For this review, take the finished solid that the model builds, in its own axes (mm). Face numbers are marked on the shaded views. Give positions to 0.01 mm unless a question says otherwise; leave off trailing zeros. Loops run counter-clockwise (first coordinate to the right, second up) from the corner with the lowest first, then second, coordinate; pieces in that order, holes last.
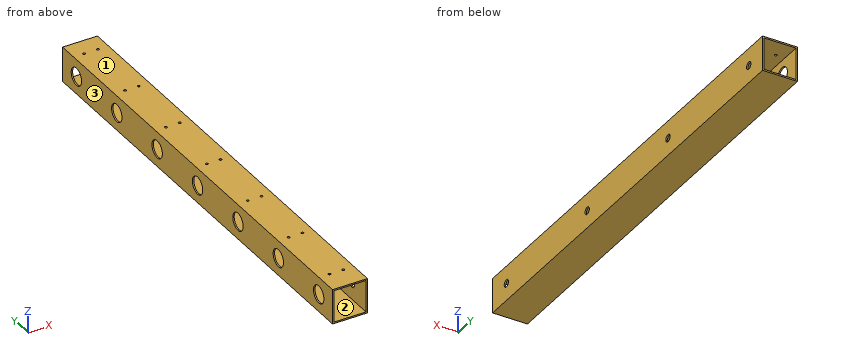
```python
from build123d import *

# Parameters (mm, degrees)
F0_W     = 76.2
F0_H     = 76.2
F0_W_2   = 69.85
F0_H_2   = 69.85
F1_DEPTH = 990.6
F2_R     = 2.75
F3_DEPTH = 25.4
F4_R     = 7.9375
F5_DEPTH = 25.4
F6_R     = 19.05
F7_DEPTH = 25.4


with BuildPart() as f1:
    # F0 (on Front) → F1 (new body)
    with BuildSketch(Plane.XZ):
        Rectangle(F0_W, F0_H)
        Rectangle(F0_W_2, F0_H_2, mode=Mode.SUBTRACT)
    extrude(amount=F1_DEPTH)

    # F2 (on face) → F3 (cut)
    with BuildSketch(Plane.XY.offset(38.1)):
        with Locations((-15.0013, -940.6)):
            Circle(F2_R)
        with Locations((14.9987, -940.6)):
            Circle(F2_R)
        with Locations((14.9987, -790.6)):
            Circle(F2_R)
        with Locations((-15.0013, -790.6)):
            Circle(F2_R)
        with Locations((14.9987, -640.6)):
            Circle(F2_R)
        with Locations((-15.0013, -640.6)):
            Circle(F2_R)
        with Locations((14.9987, -490.6)):
            Circle(F2_R)
        with Locations((-15.0013, -490.6)):
            Circle(F2_R)
        with Locations((14.9987, -340.6)):
            Circle(F2_R)
        with Locations((-15.0013, -340.6)):
            Circle(F2_R)
        with Locations((14.9987, -190.6)):
            Circle(F2_R)
        with Locations((-15.0013, -190.6)):
            Circle(F2_R)
        with Locations((14.9987, -40.6)):
            Circle(F2_R)
        with Locations((-15.0013, -40.6)):
            Circle(F2_R)
    extrude(amount=-F3_DEPTH, mode=Mode.SUBTRACT)

    # F4 (on face) → F5 (cut)
    with BuildSketch(Plane.YZ.offset(38.1)):
        with Locations((-939.8, 0)):
            Circle(F4_R)
        with Locations((-643.466667, 0)):
            Circle(F4_R)
        with Locations((-347.133333, 0)):
            Circle(F4_R)
        with Locations((-50.8, 0)):
            Circle(F4_R)
    extrude(amount=-F5_DEPTH, mode=Mode.SUBTRACT)

    # F6 (on face) → F7 (cut)
    with BuildSketch(Plane(origin=(-38.1, 0, 0), x_dir=(0, -1, 0), z_dir=(-1, 0, 0))):
        with BuildLine():
            Line((643.466667, 0), (662.516667, 0))
            ThreePointArc((662.516667, 0), (643.466667, 19.05), (624.416667, 0))
            Line((624.416667, 0), (643.466667, 0))
        make_face()
        with Locations((50.8, 0)):
            Circle(F6_R)
        with BuildLine():
            ThreePointArc((179.916667, 0), (198.966667, -19.05), (218.016667, 0))
            Line((218.016667, 0), (179.916667, 0))
        make_face()
        with BuildLine():
            Line((179.916667, 0), (218.016667, 0))
            ThreePointArc((218.016667, 0), (198.966667, 19.05), (179.916667, 0))
        make_face()
        with BuildLine():
            ThreePointArc((328.083333, 0), (347.133333, -19.05), (366.183333, 0))
            Line((366.183333, 0), (347.133333, 0))
            Line((347.133333, 0), (328.083333, 0))
        make_face()
        with BuildLine():
            Line((347.133333, 0), (366.183333, 0))
            ThreePointArc((366.183333, 0), (347.133333, 19.05), (328.083333, 0))
            Line((328.083333, 0), (347.133333, 0))
        make_face()
        with BuildLine():
            ThreePointArc((476.25, 0), (495.3, -19.05), (514.35, 0))
            Line((514.35, 0), (476.25, 0))
        make_face()
        with BuildLine():
            Line((476.25, 0), (514.35, 0))
            ThreePointArc((514.35, 0), (495.3, 19.05), (476.25, 0))
        make_face()
        with BuildLine():
            ThreePointArc((624.416667, 0), (643.466667, -19.05), (662.516667, 0))
            Line((662.516667, 0), (643.466667, 0))
            Line((643.466667, 0), (624.416667, 0))
        make_face()
        with BuildLine():
            ThreePointArc((958.85, 0), (939.8, 19.05), (920.75, 0))
            ThreePointArc((920.75, 0), (939.8, -19.05), (958.85, 0))
        make_face()
        with BuildLine():
            ThreePointArc((810.683333, 0), (791.633333, 19.05), (772.583333, 0))
            Line((772.583333, 0), (810.683333, 0))
        make_face()
        with BuildLine():
            Line((810.683333, 0), (772.583333, 0))
            ThreePointArc((772.583333, 0), (791.633333, -19.05), (810.683333, 0))
        make_face()
    extrude(amount=-F7_DEPTH, mode=Mode.SUBTRACT)


solid = f1.part
```
Item 1: Take a section at A-A on y = -846. Give the boundary of the cut face in (x, z) (3 decimals), and give its area (3 significant figures).
Answer:
outline: (-38.1, -38.1) - (38.1, -38.1) - (38.1, 38.1) - (-38.1, 38.1) - close; hole (-34.925, -34.925) - (34.925, -34.925) - (34.925, 34.925) - (-34.925, 34.925) - close
area: 927 mm2
Item 2: For L1, parallel to X at y = -940, z = 36; L2, parallel to X at y = -940.6, z = 36.9; L3, parallel to X at y = -450, z = 25 (3 decimals), list the stretches that pass through material, from the lowest coordinate up.
Answer:
L1: x = -38.1 to -17.69, -12.32 to 12.31, 17.68 to 38.1
L2: x = -38.1 to -17.75, -12.25 to 12.25, 17.75 to 38.1
L3: x = -38.1 to -34.925, 34.925 to 38.1
Item 3: The part is to be moulded in two halves that separate along X. For the marked faces 1, 2 and 3, say which applies: released by +X, released by -X, zero draft, split by the parting line, or undercut.
Answer:
face 1: zero draft
face 2: undercut
face 3: released by -X
Item 4: Clearance check with flat-ended pins moving along their axes: pin 1 Ø14.5 at (y, z) = (-50.8, 0) entering from +X; pin 2 Ø3.5 at (x, y) = (-15, -490.6) entering from +Z (3 decimals); pin 3 Ø20.5 at (y, z) = (-939.8, 0) entering from -X (3 decimals). State where each tip first meets the part, or that it passes through.
Answer:
pin 1: passes through
pin 2: stops at z = -34.925
pin 3: stops at x = 34.925
